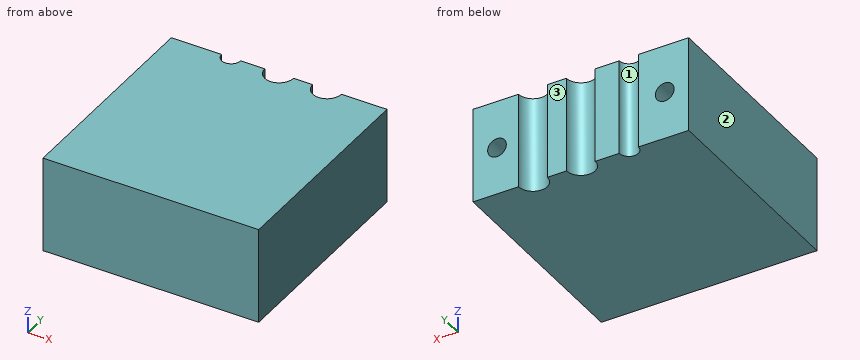
```python
from build123d import *

# Parameters (mm, degrees)
BOSS_EXTRUDE1_DEPTH = 20
SKETCH2_R           = 1.95
CUT_EXTRUDE1_DEPTH  = 20


with BuildPart() as part:
    # Sketch1 → Boss-Extrude1 (new body)
    with BuildSketch(Plane.XY):
        with BuildLine():
            Line((-22.5, -22.5), (22.5, -22.5))
            Line((22.5, -22.5), (22.5, 22.5))
            Line((22.5, 22.5), (13, 22.5))
            ThreePointArc((13, 22.5), (10, 19.5), (7, 22.5))
            Line((7, 22.5), (3, 22.5))
            ThreePointArc((3, 22.5), (0, 19.5), (-3, 22.5))
            Line((-3, 22.5), (-8, 22.5))
            ThreePointArc((-8, 22.5), (-10, 20.5), (-12, 22.5))
            Line((-12, 22.5), (-22.5, 22.5))
            Line((-22.5, 22.5), (-22.5, -22.5))
        make_face()
    extrude(amount=BOSS_EXTRUDE1_DEPTH)

    # Sketch2 → Cut-Extrude1 (cut)
    with BuildSketch(Plane(origin=(0, 22.5, 0), x_dir=(1, 0, 0), z_dir=(0, 1, 0))):
        with Locations((-17.5, -10)):
            Circle(SKETCH2_R)
        with Locations((17.5, -10)):
            Circle(SKETCH2_R)
    extrude(amount=-CUT_EXTRUDE1_DEPTH, mode=Mode.SUBTRACT)


solid = part.part
```
Can you work these out from the model? Positions are in its coordinate system, mm. Face numbers are marked on the shaded views. Coordinates: 2 decimals unless noted, no trailing zeros. Write each loop counter-clockwise with the first axis right and the second up, starting at its lowest first coordinate (ties: lowest second). Pieces come first, ordered by that corner, then holes. Notation, with made-up numbers: M 60.5,76.25 L 107.5,76.25 A19 ccw 107.5,91.25 Z; hole C 58.25,-16.5 d4. An arc over 180 degrees is marked long. Write item = value, one per line. Start each with the question number.
Q1. If we section it at B-B, the plane z = 10: Write out the boundary of the cut face in (x, y).
Q2. I'm going to push a flat-ended pin straight in: pin 1 (1.2 mm diameter, centred on x = 17, z = 11, fed in from +Y). Where does the tip first touch, or does it pass through?
Q3. If we section it at C-C, the plane x = 17.5: Write out the boundary of the cut face in (y, z), then the cut area to 3 significant figures.
Q4. Thinking about a two-plate mould opening in X: for the marked faces 1, 2 and 3, which applies, released by +X, released by -X, zero draft, split by the parting line, or undercut?
Q5. If I drill on L1, parallel to X at y = 11.5, z = 10; L2, parallel to Z at x = -17.5, y = 10.5; L3, parallel to Y at x = 16, z = 9.25, over which ranges is the centre line in solid material (lowest first)? Write a range as [from, to].
Q6. If we section it at A-A, the plane y = 15.5: Write out the boundary of the cut face in (x, z), then the cut area to 3 significant figures.
Q7. If we section it at D-D, the plane z = 3.75: Write out the boundary of the cut face in (x, y).
Check sheet entries:
q1.outline = M -22.5,-22.5 L 22.5,-22.5 L 22.5,22.5 L 19.45,22.5 L 19.45,2.5 L 15.55,2.5 L 15.55,22.5 L 13,22.5 A3 cw 7,22.5 L 3,22.5 A3 cw -3,22.5 L -8,22.5 A2 cw -12,22.5 L -15.55,22.5 L -15.55,2.5 L -19.45,2.5 L -19.45,22.5 L -22.5,22.5 Z
q2.pin_1 = 2.5
q3.outline = M -22.5,0 L 22.5,0 L 22.5,8.05 L 2.5,8.05 L 2.5,11.95 L 22.5,11.95 L 22.5,20 L -22.5,20 Z
q3.area = 822 mm²
q4.face_1 = undercut
q4.face_2 = released by -X
q4.face_3 = zero draft
q5.L1 = [-22.5, -19.45], [-15.55, 15.55], [19.45, 22.5]
q5.L2 = [0, 8.05], [11.95, 20]
q5.L3 = [-22.5, 2.5]
q6.outline = M -22.5,0 L 22.5,0 L 22.5,20 L -22.5,20 Z; hole C -17.5,10 d3.9; hole C 17.5,10 d3.9
q6.area = 876 mm²
q7.outline = M -22.5,-22.5 L 22.5,-22.5 L 22.5,22.5 L 13,22.5 A3 cw 7,22.5 L 3,22.5 A3 cw -3,22.5 L -8,22.5 A2 cw -12,22.5 L -22.5,22.5 Z
